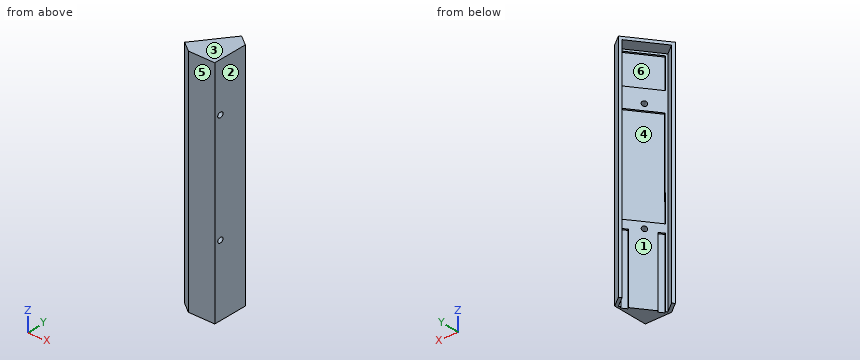
Autodesk Fusion 360 part; units mm, degrees
sketch "スケッチ1" plane through (0, 0, 0) normal (0, 0, 1) x (1, 0, 0)
  line L0 (0, 0) -> (0, 16)
  line L1 (0, 0) -> (-12, 0)
  line L2 (-12, 0) -> (0, 16)
  line L3 (0, 16) -> (0.9, 17.2)
  line L4 (-12, 0) -> (-12.5407, 0)
  line L5 (-12, 0) -> (-12.9, -1.2)
  line L6 (-12, 0) -> (-17.6, 4.2)
  line L7 (-17.6, 4.2) -> (-18.5, 3)
  line L8 (-18.5, 3) -> (-12.9, -1.2)
  line L9 (0, 16) -> (-5.6, 20.2)
  line L10 (-5.6, 20.2) -> (-4.7, 21.4)
  line L11 (-4.7, 21.4) -> (0.9, 17.2)
  line L12 (0.9, 17.2) -> (0.9, -4)
  line L13 (-12.9, -1.2) -> (1.7279, -1.2)
  dimension "d1" = 16
  dimension "d3" = 1.5
  dimension "d4" = 1.5
  dimension "d5" = 7
  dimension "d6" = 1.5
  dimension "d7" = 7
  dimension "d8" = 1.5
extrude "押し出し1" add sketch "スケッチ1" along normal blind 120
sketch "スケッチ2" plane through (-7.68, 5.76, 0) normal (-0.8, 0.6, 0) x (0, 0, 1)
  line L0 (0, 12.8) -> (0, -7.2)
  line L1 (0, -7.2) -> (120, -7.2)
  line L2 (120, -7.2) -> (120, 12.8)
  line L3 (120, 12.8) -> (0, 12.8)
  line L4 (120, 12.8) -> (118.5, 12.8)
  line L5 (118.5, 12.8) -> (118.5, -7.2)
  line L6 (118.5, -7.2) -> (120, -7.2)
  line L7 (120, -7.2) -> (120, 12.8)
  dimension "d11" = 1.5
  dimension "d12" = 20
extrude "押し出し2" add sketch "スケッチ2" along normal blind 7 contours L1 L2 L3 L4 L5 L6 L7
sketch "スケッチ3" plane through (-7.68, 5.76, 0) normal (-0.8, 0.6, 0) x (0, 0, 1)
  line L0 (118.5, -7.2) -> (118.5, 12.8)
  line L1 (118.5, 12.8) -> (0, 12.8)
  line L2 (0, 12.8) -> (0, -7.2)
  line L3 (0, -7.2) -> (118.5, -7.2)
  line L4 (118.5, -7.2) -> (94.5, -7.2)
  line L5 (94.5, -7.2) -> (94.5, 2.3)
  circle A0 centre (94.5, 2.3) radius 1.3
  line L6 (94.5, 2.3) -> (37, 2.3)
  circle A1 centre (37, 2.3) radius 1.3
  dimension "d15" = 24
  dimension "d16" = 9.5
  dimension "d17" = 2.6
  dimension "d18" = 57.5
  dimension "d19" = 2.6
extrude "押し出し3" cut sketch "スケッチ3" against normal blind 20 contours A1 | L5 A0 L6 | L5 A0 L6
sketch "スケッチ4" plane through (-7.68, 5.76, 0) normal (-0.8, 0.6, 0) x (0, 0, 1)
  circle A0 centre (37, 2.3) radius 1.3
  circle A1 centre (94.5, 2.3) radius 1.3
  line L0 (118.5, -7.2) -> (118.5, 12.8)
  line L1 (118.5, 12.8) -> (0, 12.8)
  line L2 (0, 12.8) -> (0, -7.2)
  line L3 (0, -7.2) -> (118.5, -7.2)
  line L4 (0, 12.8) -> (0, 11.8)
  line L5 (0, 11.8) -> (36, 11.8)
  line L6 (36, 11.8) -> (36, 8.8)
  line L7 (36, 8.8) -> (0, 8.8)
  line L8 (0, 8.8) -> (0, 11.8)
  line L9 (0, -7.2) -> (0, -6.2)
  line L10 (0, -6.2) -> (36, -6.2)
  line L11 (36, -6.2) -> (36, -3.2)
  line L12 (36, -3.2) -> (0, -3.2)
  line L13 (0, -3.2) -> (0, -6.2)
  line L14 (36, 11.8) -> (94, 11.8)
  line L15 (36, -6.2) -> (94, -6)
  circle A2 centre (37, 2.3) radius 3.3
  line L16 (40.2999, 2.3211) -> (40.2394, 11.8)
  line L17 (40.2697, 2.7464) -> (40.3005, -6.1852)
  circle A3 centre (94.5, 2.3) radius 3.3
  line L18 (91.2005, 2.2398) -> (91.2305, -6.4364)
  line L19 (91.2005, 2.2398) -> (91.2155, 12.5754)
  dimension "d22" = 1
  dimension "d23" = 3
  dimension "d24" = 1
  dimension "d25" = 3
  dimension "d26" = 2
  dimension "d27" = 2
extrude "押し出し4" cut sketch "スケッチ4" against normal blind 1 contours L2 L10 L11 L12 L13 | L2 L5 L6 L7 L8 | L14 L15 A2 L16 L17 L18 L19
sketch "スケッチ5" plane through (-7.68, 5.76, 0) normal (-0.8, 0.6, 0) x (0, 0, 1)
  line L0 (36, 8.8) -> (0, 8.8)
  line L1 (0, 8.8) -> (0, -3.2)
  line L2 (0, -3.2) -> (36, -3.2)
  line L3 (36, -3.2) -> (36, -6.2)
  line L4 (36, -6.2) -> (0, -6.2)
  line L5 (0, -6.2) -> (0, -7.2)
  line L6 (0, -7.2) -> (118.5, -7.2)
  line L7 (118.5, -7.2) -> (118.5, 12.8)
  line L8 (118.5, 12.8) -> (0, 12.8)
  line L9 (0, 12.8) -> (0, 11.8)
  line L10 (0, 11.8) -> (36, 11.8)
  line L11 (36, 11.8) -> (36, 8.8)
  line L12 (40.2394, 11.8) -> (91.2144, 11.8)
  line L13 (91.2144, 11.8) -> (91.2007, 2.3697)
  arc A0 (91.2007, 2.3697) -> (91.2005, 2.2398) centre (94.5, 2.3) ccw
  line L14 (91.2005, 2.2398) -> (91.229, -6.0096)
  line L15 (91.229, -6.0096) -> (40.3005, -6.1852)
  line L16 (40.3005, -6.1852) -> (40.2727, 1.8761)
  arc A1 (40.2727, 1.8761) -> (40.2999, 2.3211) centre (37, 2.3) ccw
  line L17 (40.2999, 2.3211) -> (40.2394, 11.8)
  circle A2 centre (37, 2.3) radius 1.3
  circle A3 centre (94.5, 2.3) radius 1.3
  line L18 (37, 11.8) -> (37, 7.8)
  line L19 (37, 7.8) -> (1, 7.8)
  line L20 (1, 7.8) -> (1, -2.2)
  line L21 (1, -2.2) -> (37, -2.2)
  line L22 (37, -2.2) -> (37, -6.2)
  line L23 (37, -6.2) -> (117.5, -6.2)
  line L24 (117.5, -6.2) -> (117.5, 11.8)
  line L25 (117.5, 11.8) -> (37, 11.8)
  line L26 (101.4988, 11.8) -> (101.4988, -6.2)
  dimension "d30" = -1
extrude "押し出し5" cut sketch "スケッチ5" against normal blind 1 contours L23 L24 L25 L26
Input: part model. Units: mm. Frame: model coordinates. Face numbers are marked on the shaded views. A direction names the side the tool comes from. Round coordinates to 2 decimals unless told otherwise and drop trailing zeros. Loops run counter-clockwise (first coordinate to the right, second up) from the corner with the lowest first, then second, coordinate; pieces in that order, holes last. Notation, with made-up numbers: (-19.5, -14.5) -> (-5.5, -14.5) arc R18 ccw to (-5.5, 15.5) -> close; hole circle Ø7 at (2.25, 60.25). An arc over 180 degrees is marked (long way). Use one line per item in the form item = value. Start each with the question number.
Item 1: Section query A-A on z = 98.5. Return the cut outline in (x, y).
Item 2: Section query C-C on x = -15.25. Return the cut outline in (y, z), then the cut area to 3 significant figures.
Item 3: Section query B-B on z = 13. Return the cut outline in (x, y).
Item 4: Material intervals for L1, parallel to Z at x = -7.5, y = 7; L2, parallel to X at y = 0.5, z = 75 (3 decimals); L3, parallel to X at y = 3, z = 41, sorted ascending. Write a range as from..to.
Item 5: Mould query, pull axis Z, two halves, no side actions, for the marked faces 3, 4, 5 and 6. Classes: pulls with the +Z half, pulls with the -Z half, needs draft (parallel to the pull), parting line crosses it, or undercut.
Item 6: Contact query for flat-ended pins moving along their axis: pin 1 Ø6 at (y, z) = (15.5, 21.5) entering from -X; pin 2 Ø3 at (y, z) = (8, 57.5) entering from -X (3 decimals). Output: stop coordinate, or through.
Item 7: Set-up query: the marked faces 1 and 2. Return all of +Z, -Z, +X, -X, +Y, -Y with unobstructed straight access to the full face (end or side cutting, diameter ignored); none if empty.
Item 8: Section query D-D on z = 49. Return the cut outline in (x, y).
Ans:
q1.outline = (-18.5, 3) -> (-12.9, -1.2) -> (0.9, -1.2) -> (0.9, 17.2) -> (-4.7, 21.4) -> (-5.6, 20.2) -> (0, 16) -> (-12, 0) -> (-17.6, 4.2) -> close
q2.outline = (0.56, 0) -> (2.44, 0) -> (2.44, 118.5) -> (7.33, 118.5) -> (7.33, 120) -> (0.56, 120) -> close
q2.area = 232 mm^2
q3.outline = (-18.5, 3) -> (-12.9, -1.2) -> (0.9, -1.2) -> (0.9, 17.2) -> (-4.7, 21.4) -> (-5.6, 20.2) -> (0, 16) -> (-0.6, 15.2) -> (0.2, 14.6) -> (-1.6, 12.2) -> (-2.4, 12.8) -> (-9.6, 3.2) -> (-8.8, 2.6) -> (-10.6, 0.2) -> (-11.4, 0.8) -> (-12, 0) -> (-17.6, 4.2) -> close
q4.L1 = 118.5..120
q4.L2 = -15.167..-12.667, -11.625..-10.776, -10.375..0.9
q4.L3 = -18.5..-16, -8.5..0.9
q5.face_3 = pulls with the +Z half
q5.face_4 = undercut
q5.face_5 = needs draft
q5.face_6 = undercut
q6.pin_1 = -3.33
q6.pin_2 = -5.875
q7.face_1 = -Z
q7.face_2 = +Z, -Z, +X, +Y, -Y
q8.outline = (-18.5, 3) -> (-12.9, -1.2) -> (0.9, -1.2) -> (0.9, 17.2) -> (-4.7, 21.4) -> (-5.6, 20.2) -> (0, 16) -> (-0.6, 15.2) -> (0.2, 14.6) -> (-10.57, 0.24) -> (-11.37, 0.84) -> (-12, 0) -> (-17.6, 4.2) -> close
